from build123d import *

# Parameters (mm, degrees)
SKETCH1_R                  = 57
EXTRUDE4_DEPTH             = 7.5
SKETCH_R                   = 60
SKETCH_R_2                 = 57
EXTRUDE5_DEPTH             = 5
EXTRUDE6_DEPTH             = 86.183625187
EXTRUDE6_DEPTH_BACK        = 86.183625187
SKETCH5_R                  = 18
F_4_5_4_5_DIAMETER_HOLE1_D = 4.5
CIRPATTERN1_COUNT          = 4
M5_CLEARANCE_HOLE1_D       = 5.5
M8_CLEARANCE_HOLE2_D       = 9
CIRPATTERN3_COUNT          = 4


with BuildPart() as part:
    # Sketch1 → Extrude4 (new, symmetric)
    with BuildSketch(Plane(origin=(0, 0, 0), x_dir=(1, 0, 0), z_dir=(0, 1, 0))):
        with Locations(Location((0, 0, 0), (0, 0, 270))):
            Circle(SKETCH1_R)
    extrude(amount=EXTRUDE4_DEPTH, both=True)

    # Sketch → Extrude5 (add, symmetric)
    with BuildSketch(Plane(origin=(0, 0, 0), x_dir=(1, 0, 0), z_dir=(0, 1, 0))):
        with Locations(Location((0, 0, 0), (0, 0, 270))):
            Circle(SKETCH_R)
        with Locations(Location((0, 0, 0), (0, 0, 270))):
            Circle(SKETCH_R_2, mode=Mode.SUBTRACT)
    extrude(amount=EXTRUDE5_DEPTH, both=True)

    # Sketch5 → Extrude6 (cut, two sides: drawn at the far end of the back side and taken through both)
    with BuildSketch(Plane(origin=(0, 0, 0), x_dir=(1, 0, 0), z_dir=(0, 1, 0)).offset(-EXTRUDE6_DEPTH_BACK)):
        with Locations(Location((0, 0, 0), (0, 0, 270))):
            Circle(SKETCH5_R)
    extrude(amount=EXTRUDE6_DEPTH + EXTRUDE6_DEPTH_BACK, mode=Mode.SUBTRACT)

    # 4.5 _4.5_ Diameter Hole1 (through all)
    with Locations(Plane(origin=(0, -7.5, 0), x_dir=(-1, 0, 0), z_dir=(0, -1, 0))):
        with Locations((15.556349186, 15.556349186)):
            f_4_5_4_5_diameter_hole1 = Hole(F_4_5_4_5_DIAMETER_HOLE1_D / 2)

    # CirPattern1: 4.5 _4.5_ Diameter Hole1 ×4 about axis
    cirpattern1_axis = Axis((0, 0, 0), (0, 1, 0))
    for i in range(1, CIRPATTERN1_COUNT):
        add(f_4_5_4_5_diameter_hole1.rotate(cirpattern1_axis, i * 360 / CIRPATTERN1_COUNT), mode=Mode.SUBTRACT)

    # M5 Clearance Hole1 (through all)
    with Locations(Plane(origin=(0, 7.5, 0), x_dir=(1, 0, 0), z_dir=(0, 1, 0))):
        with Locations((-37.5, 18), (-37.5, -18), (37.5, -18), (37.5, 18)):
            Hole(M5_CLEARANCE_HOLE1_D / 2)

    # M8 Clearance Hole2 (through all)
    with Locations(Plane(origin=(0, 7.5, 0), x_dir=(1, 0, 0), z_dir=(0, 1, 0))):
        with Locations((-35.355339059, -35.355339059)):
            m8_clearance_hole2 = Hole(M8_CLEARANCE_HOLE2_D / 2)

    # CirPattern3: M8 Clearance Hole2 ×4 about axis
    cirpattern3_axis = Axis((0, 0, 0), (0, 1, 0))
    for i in range(1, CIRPATTERN3_COUNT):
        add(m8_clearance_hole2.rotate(cirpattern3_axis, i * 360 / CIRPATTERN3_COUNT), mode=Mode.SUBTRACT)


solid = part.part
The listing builds one solid part. Answer for the finished solid, in the listing's coordinates (mm). A direction names the side the tool comes from. Round coordinates to 2 decimals unless told otherwise and drop trailing zeros. Order: outer loops, then holes, each group sorted by start corner. A loop starts at its lowest first (then second) coordinate and runs counter-clockwise, first axis right, second up. Notation, with made-up numbers: (-2, 58) -> (20, 58) arc R9 cw to (20, 62) -> close; hole circle Ø2 at (64, -8.75). An arc over 180 degrees is marked (long way). One line per item, written item: value.
Item 1: For a pull along Z with two mould halves and no side action, classify faces 1 (the flat face through (13, -7.5, -13)), 2 (the cylindrical face through (-55.645, -6.232, -12.356)), 3 (the cylindrical face through (16.04, 0.1, 13.36)) as released by +Z, released by -Z, zero draft, split by the parting line, or undercut.
Taken from the geometry:
face 1: zero draft
face 2: split by the parting line
face 3: undercut
Item 2: Find section C-C, the plane x = 37.5. Give the vertices of the cut face in (y, z).
Taken from the geometry:
outline: (-7.5, -42.93) -> (-5, -42.93) -> (-5, -46.84) -> (5, -46.84) -> (5, -42.93) -> (7.5, -42.93) -> (7.5, -39.31) -> (-7.5, -39.31) -> close; (-7.5, -31.4) -> (7.5, -31.4) -> (7.5, -20.75) -> (-7.5, -20.75) -> close; (-7.5, -15.25) -> (7.5, -15.25) -> (7.5, 15.25) -> (-7.5, 15.25) -> close; (-7.5, 20.75) -> (7.5, 20.75) -> (7.5, 31.4) -> (-7.5, 31.4) -> close; (-7.5, 39.31) -> (7.5, 39.31) -> (7.5, 42.93) -> (5, 42.93) -> (5, 46.84) -> (-5, 46.84) -> (-5, 42.93) -> (-7.5, 42.93) -> close
Item 3: Find section A-A, the plane x = 0. Give the vertices of the cut face in (y, z).
Taken from the geometry:
outline: (-7.5, -57) -> (-5, -57) -> (-5, -60) -> (5, -60) -> (5, -57) -> (7.5, -57) -> (7.5, -18) -> (-7.5, -18) -> close; (-7.5, 18) -> (7.5, 18) -> (7.5, 57) -> (5, 57) -> (5, 60) -> (-5, 60) -> (-5, 57) -> (-7.5, 57) -> close
Item 4: Given P1, Ø9, axis at x = 37.5, z = 18, coming from the -Y side; P2, Ø7, axis at x = 35.36, z = 35.36, coming from the +Y side; P3, Ø1, axis at y = -4, z = -25, coming from the -X side; P4, Ø1.5, axis at x = 38, y = 1, coming from the -Z side, each flat-ended and moving along its own axis, determine where each tip first touches the part or whether it passes through.
Taken from the geometry:
P1: stops at y = -7.5
P2: passes through
P3: stops at x = -54.77
P4: stops at z = -47.04
Item 5: Find section D-D, the plane z = -44. Give the vertices of the cut face in (x, y).
Taken from the geometry:
outline: (-40.79, -5) -> (-36.24, -5) -> (-36.24, -7.5) -> (36.24, -7.5) -> (36.24, -5) -> (40.79, -5) -> (40.79, 5) -> (36.24, 5) -> (36.24, 7.5) -> (-36.24, 7.5) -> (-36.24, 5) -> (-40.79, 5) -> close
Item 6: Find section B-B, the plane z = 0. Give the vertices of the cut face in (x, y).
Taken from the geometry:
outline: (-60, -5) -> (-57, -5) -> (-57, -7.5) -> (-18, -7.5) -> (-18, 7.5) -> (-57, 7.5) -> (-57, 5) -> (-60, 5) -> close; (18, -7.5) -> (57, -7.5) -> (57, -5) -> (60, -5) -> (60, 5) -> (57, 5) -> (57, 7.5) -> (18, 7.5) -> close
Item 7: For faces 4 (the flat face through (-22, 5, 53)), 5 (the flat face through (-22, -5, 53)), 6 (the cylindrical face through (5.407, -0.105, 17.169)), determine the directions among +Z, -Z, +X, -X, +Y, -Y from which every point of the face is accessible in a straight line to the end or side of a thin tool.
Taken from the geometry:
face 4: +Y
face 5: -Y
face 6: +Y, -Y
Item 8: Straight lines are drawn through the part: L1, parallel to X at y = 3, z = 0; L2, parallel to Z at x = -34, y = -2.5; L3, parallel to Z at x = 13.5, y = -2. For each, find the intervals that lie inside material, in ascending order.
Taken from the geometry:
L1: x = -60 to -18, 18 to 60
L2: z = -49.44 to -39.65, -31.06 to 31.06, 39.65 to 49.44
L3: z = -58.46 to -16.47, -14.64 to -11.91, 11.91 to 14.64, 16.47 to 58.46
